Build history of the part. All positions in model axes, mm. Coordinates: 2 decimals unless noted, no trailing zeros. Write each loop counter-clockwise with the first axis right and the second up, starting at its lowest first coordinate (ties: lowest second). Pieces come first, ordered by that corner, then holes.
from build123d import *

# Parameters (mm, degrees)
SKETCH1_W           = 495.3
SKETCH1_H           = 57.15
BOSS_EXTRUDE1_DEPTH = 3.175
SKETCH23_W          = 495.3
SKETCH23_H          = 381.64999997
BOSS_EXTRUDE3_DEPTH = 3.175
SKETCH24_W          = 88.9
SKETCH24_H          = 63.5
SKETCH24_W_2        = 139.7
SKETCH24_W_3        = 82.55
CUT_EXTRUDE6_DEPTH  = 6.35
CUT_EXTRUDE7_DEPTH  = 6.35
SKETCH27_W          = 279.4
SKETCH27_H          = 25.4
CUT_EXTRUDE8_DEPTH  = 6.35


with BuildPart() as part:
    # Sketch1 → Boss-Extrude1 (new, symmetric)
    with BuildSketch(Plane(origin=(0, 0, 0), x_dir=(1, 0, 0), z_dir=(0, 1, 0))):
        Rectangle(SKETCH1_W, SKETCH1_H)
    extrude(amount=BOSS_EXTRUDE1_DEPTH, both=True)

    # Sketch23 → Boss-Extrude3 (add, symmetric)
    with BuildSketch(Plane(origin=(0, 0, 0), x_dir=(1, 0, 0), z_dir=(0, 1, 0))):
        with Locations((-0.01297497, 0)):
            Rectangle(SKETCH23_W, SKETCH23_H)
    extrude(amount=BOSS_EXTRUDE3_DEPTH, both=True)

    # Sketch24 → Cut-Extrude6 (cut)
    with BuildSketch(Plane(origin=(0, 3.175, 0), x_dir=(1, 0, 0), z_dir=(0, 1, 0))):
        with Locations((203.18702503, -159.074999985)):
            Rectangle(SKETCH24_W, SKETCH24_H)
        with Locations((-6.36297497, -159.074999985)):
            Rectangle(SKETCH24_W_2, SKETCH24_H)
        with Locations((-206.38797497, -159.074999985)):
            Rectangle(SKETCH24_W_3, SKETCH24_H)
    extrude(amount=-CUT_EXTRUDE6_DEPTH, mode=Mode.SUBTRACT)

    # Sketch25 → Cut-Extrude7 (cut)
    with BuildSketch(Plane(origin=(0, 3.175, 0), x_dir=(1, 0, 0), z_dir=(0, 1, 0))):
        with BuildLine():
            Line((114.28702503, -89.224999985), (114.28702503, -178.124999985))
            ThreePointArc((114.28702503, -178.124999985), (111.11202503, -181.299999985), (107.93702503, -178.124999985))
            Line((107.93702503, -178.124999985), (107.93702503, -89.224999985))
            ThreePointArc((107.93702503, -89.224999985), (111.11202503, -86.049999985), (114.28702503, -89.224999985))
        make_face()
        with BuildLine():
            Line((-117.48797497, -89.224999985), (-117.48797497, -178.124999985))
            ThreePointArc((-117.48797497, -178.124999985), (-120.66297497, -181.299999985), (-123.83797497, -178.124999985))
            Line((-123.83797497, -178.124999985), (-123.83797497, -89.224999985))
            ThreePointArc((-123.83797497, -89.224999985), (-120.66297497, -86.049999985), (-117.48797497, -89.224999985))
        make_face()
    extrude(amount=-CUT_EXTRUDE7_DEPTH, mode=Mode.SUBTRACT)

    # Sketch27 → Cut-Extrude8 (cut)
    with BuildSketch(Plane(origin=(0, 3.175, 0), x_dir=(1, 0, 0), z_dir=(0, 1, 0))):
        with Locations((-107.96297497, 178.124999985)):
            Rectangle(SKETCH27_W, SKETCH27_H)
    extrude(amount=-CUT_EXTRUDE8_DEPTH, mode=Mode.SUBTRACT)


solid = part.part
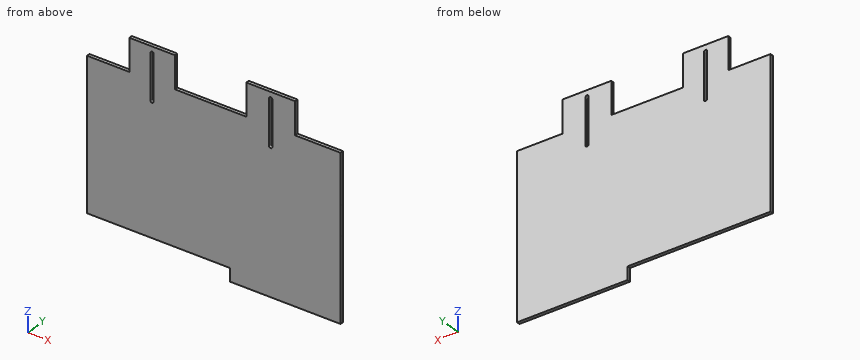
(1) Slice it at B-B, the plane y = -2. List the corners of the cut face in (x, z) (3 decimals).
(2) Slice it at D-D, the plane x = -111.5. List the corners of the cut face in (y, z) (3 decimals).
(3) Slice it at A-A, the plane z = 148.5. List the corners of the cut face in (x, y) (3 decimals).
(4) Flat gauge pins, fed straight in: P1, Ø1.9, axis at y = 0, z = 166.5, coming from the +X side; P2, Ø2, axis at y = 0, z = 67, coming from the +X side; P3, Ø1.9, axis at y = 1.5, z = 170, coming from the -X side. Where does each tip first touch, or does it go through?
(5) Slice it at C-C, the plane x = 183. List the corners of the cut face in (y, z) (3 decimals), and give its area (3 significant figures).
(6) Probe L1, parallel to X at y = -0.5, z = 110; L2, parallel to X at y = -2.5, z = 155; L3, parallel to X at y = 1.25, z = -142. List the from-to ranges inside material, lowest first.
Results:
1. outline: (-247.663, -165.425) - (31.737, -165.425) - (31.737, -190.825) - (247.637, -190.825) - (247.637, -28.575) - (247.65, -28.575) - (247.65, 28.575) - (247.637, 28.575) - (247.637, 127.325) - (158.737, 127.325) - (158.737, 190.825) - (63.487, 190.825) - (63.487, 127.325) - (-76.213, 127.325) - (-76.213, 190.825) - (-165.113, 190.825) - (-165.113, 127.325) - (-247.663, 127.325) - close; hole (-123.838, 89.225) arc R3.175 ccw to (-117.488, 89.225) - (-117.488, 178.125) arc R3.175 ccw to (-123.838, 178.125) - close; hole (107.937, 89.225) arc R3.175 ccw to (114.287, 89.225) - (114.287, 178.125) arc R3.175 ccw to (107.937, 178.125) - close
2. outline: (-3.175, -165.425) - (3.175, -165.425) - (3.175, 190.825) - (-3.175, 190.825) - close
3. outline: (-165.113, -3.175) - (-123.838, -3.175) - (-123.838, 3.175) - (-165.113, 3.175) - close; (-117.488, -3.175) - (-76.213, -3.175) - (-76.213, 3.175) - (-117.488, 3.175) - close; (63.487, -3.175) - (107.937, -3.175) - (107.937, 3.175) - (63.487, 3.175) - close; (114.287, -3.175) - (158.737, -3.175) - (158.737, 3.175) - (114.287, 3.175) - close
4. P1: stops at x = 158.74
4. P2: stops at x = 247.64
4. P3: stops at x = -165.11
5. outline: (-3.175, -190.825) - (3.175, -190.825) - (3.175, 127.325) - (-3.175, 127.325) - close
5. area: 2,020 mm2
6. L1: x = -247.66 to -123.84, -117.49 to 107.94, 114.29 to 247.64
6. L2: x = -165.11 to -123.84, -117.49 to -76.21, 63.49 to 107.94, 114.29 to 158.74
6. L3: x = -247.66 to 247.64
